Build history of the part. All positions in model axes, mm. Face numbers are marked on the shaded views. A direction names the side the tool comes from. Give positions to 0.01 mm unless a question says otherwise; leave off trailing zeros. Write each loop counter-clockwise with the first axis right and the second up, starting at its lowest first coordinate (ties: lowest second). Pieces come first, ordered by that corner, then holes. Notation, with made-up numbers: M 6.5,-21.5 L 53.5,-21.5 A22 cw 53.5,4.5 Z; hole C 40,-29 d6. An arc over 180 degrees is marked long. Return JSON: item names as keys, results as strings. Group by question number.
Q1. Wall check: probe 1 along Y at (x, z) = (-30.5, 357); probe 2 along Z at (x, y) = (56.5, 82.5); probe 3 along X at (y, z) = (91.5, 218). Give the ranges that are in metal, low to high.
Q2. Band-saw the part on D-D, the plane z = 142. Give the cut face in (x, y), then the cut area to 3 significant figures.
Q3. Tool access for the marked faces 1, 2 and 3: list every direction of +Z, -Z, +X, -X, +Y, -Y with a clear straight run to the whole face (end or side of a thin tool).
Q4. Flat gauge pins, fed straight in: pin 1 Ø8 at (y, z) = (-61.5, 146.5) entering from -X; pin 2 Ø25 at (y, z) = (-96, 302.5) entering from +X. Where does each tip first touch, or does it go through?
Q5. Band-saw the part on A-A, the plane z = 352. Give the cut face in (x, y), then the cut area to 3 significant figures.
Q6. Pull direction Y, two halves, no side cores. Call the marked faces 4, 5, 6 and 7: +Y half, -Y half, draft (parallel to the pull), parting line (faces both ways), or undercut.
Q7. Band-saw the part on C-C, the plane y = 85.5. Give the cut face in (x, z).
Q8. Band-saw the part on B-B, the plane x = 0. Give the cut face in (y, z), then the cut area to 3 significant figures.
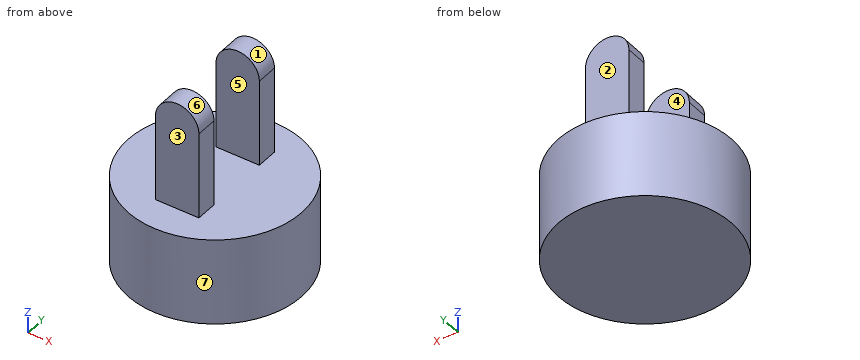
from build123d import *

# Parameters (mm, degrees)
SKETCH1_R           = 200
BOSS_EXTRUDE1_DEPTH = 200
BOSS_EXTRUDE2_START = 75
BOSS_EXTRUDE2_DEPTH = 50
BOSS_EXTRUDE3_START = -125
BOSS_EXTRUDE3_DEPTH = 50


with BuildPart() as part:
    # Sketch1 → Boss-Extrude1 (new body)
    with BuildSketch(Plane.XY):
        Circle(SKETCH1_R)
    extrude(amount=BOSS_EXTRUDE1_DEPTH)

    # Sketch2 → Boss-Extrude2 (add)
    with BuildSketch(Plane(origin=(0, 0, 0), x_dir=(1, 0, 0), z_dir=(0, 1, 0)).offset(BOSS_EXTRUDE2_START)):
        with BuildLine():
            Line((-50, -200), (-50, -400))
            ThreePointArc((-50, -400), (0, -450), (50, -400))
            Line((50, -400), (50, -200))
            Line((50, -200), (-50, -200))
        make_face()
    extrude(amount=BOSS_EXTRUDE2_DEPTH)

    # Sketch2<2> → Boss-Extrude3 (add)
    with BuildSketch(Plane(origin=(0, 0, 0), x_dir=(1, 0, 0), z_dir=(0, 1, 0)).offset(BOSS_EXTRUDE3_START)):
        with BuildLine():
            Line((-50, -200), (-50, -400))
            ThreePointArc((-50, -400), (0, -450), (50, -400))
            Line((50, -400), (50, -200))
            Line((50, -200), (-50, -200))
        make_face()
    extrude(amount=BOSS_EXTRUDE3_DEPTH)


solid = part.part
From the geometry:
{
 "1": {"probe 1": "y = -125 to -75, 75 to 125", "probe 2": "z = 0 to 200", "probe 3": "x = -50 to 50"},
 "2": {"outline": "C 0,0 d400", "area": "126,000 mm^2"},
 "3": {"face 1": "+Z, +Y, -Y", "face 2": "+Z, +X, -X, +Y", "face 3": "+Z, +X, -X, -Y"},
 "4": {"pin 1": "stops at x = -191.56", "pin 2": "stops at x = 50"},
 "5": {"outline": "M -50,-125 L 50,-125 L 50,-75 L -50,-75 Z; M -50,75 L 50,75 L 50,125 L -50,125 Z", "area": "10,000 mm^2"},
 "6": {"face 4": "undercut", "face 5": "undercut", "face 6": "draft", "face 7": "parting line"},
 "7": {"outline": "M -180.8,0 L 180.8,0 L 180.8,200 L 50,200 L 50,400 A50 ccw -50,400 L -50,200 L -180.8,200 Z"},
 "8": {"outline": "M -200,0 L 200,0 L 200,200 L 125,200 L 125,450 L 75,450 L 75,200 L -75,200 L -75,450 L -125,450 L -125,200 L -200,200 Z", "area": "105,000 mm^2"}
}
